Work out the finished part from the listing and answer in its coordinate system (mm). A direction names the side the tool comes from. Give positions to 0.01 mm unless a question says otherwise; leave off trailing zeros. Write each loop counter-clockwise with the first axis right and the second up, starting at its lowest first coordinate (ties: lowest second). Pieces come first, ordered by that corner, then holes. Notation, with made-up numbers: (31, 22.25) -> (56, 22.25) arc R32 cw to (56, 54.25) -> close; hole circle Ø1 at (87.5, -38.75). An arc over 180 degrees is marked (long way). Use a Markdown table: item, result. Add a question column.
Q1. For faces 1 (the face through (0, 0, 76.2)), 2 (the face through (0, -22, 12.7)), determine the directions among +Z, -Z, +X, -X, +Y, -Y from which every point of the face is accessible in a straight line to the end or side of a thin tool.
Q2. Section A-A, the plane z = 27.5 is taken. Give the vertices of the cut face in (x, y), plus the area to 3 significant figures.
Q3. Each of these flat-tipped pins is pushed along its axis until it touches: pin 1 Ø1 at (y, z) = (-29, 11) entering from +X; pin 2 Ø10 at (y, z) = (26.5, 9.5) entering from +X; pin 3 Ø2 at (x, y) = (-20.5, -16) entering from +Z; pin 4 Ø1 at (y, z) = (-16.5, 21) entering from -X. Where does it stop, or does it pass through?
Q4. Section B-B, the plane z = 67 is taken. Give the vertices of the cut face in (x, y), plus the area to 3 significant figures.
Q5. Consider line 1 (Z direction, x = -21, y = 7); line 2 (Y direction, x = 7, z = 37); line 3 (X direction, y = 5.5, z = 14). Determine where each line is inside the solid, lowest interval first.
from build123d import *

# Parameters (mm, degrees)
F0_R     = 38.1
F1_DEPTH = 12.7
F4_R     = 5.08


with BuildPart() as f1:
    # F0 (on Top) → F1 (new body)
    with BuildSketch(Plane.XY):
        Circle(F0_R)
    extrude(amount=F1_DEPTH)

    # F2 (on Front) → F3 (revolve)
    with BuildSketch(Plane.XZ):
        Polygon((0, 69.85), (0, 12.7), (16.740909, 12.7), (6.35, 69.85), (6.35, 76.2), (0, 76.2), align=None)
    revolve(axis=Axis((0, 0, 41.275), (0, 0, 1)))

    # F4
    f4_edges = [f1.edges().sort_by_distance(p)[0] for p in [
        (-38.1, 0, 12.7),
        (-38.1, 0, 0),
        (-6.35, 0, 76.2),
        (-16.740909, 0, 12.7),
    ]]
    fillet(f4_edges, radius=F4_R)


solid = f1.part
Result set:
| question | item | result |
|---|---|---|
| 1 | face 1 | +Z, +X, -X, +Y, -Y |
| 1 | face 2 | +Z |
| 2 | outline | circle Ø28.1 at (0, 0) |
| 2 | area | 620 mm2 |
| 3 | pin 1 | stops at x = 23.58 |
| 3 | pin 2 | stops at x = 31.3 |
| 3 | pin 3 | stops at z = 12.7 |
| 3 | pin 4 | passes through |
| 4 | outline | circle Ø13.74 at (0, 0) |
| 4 | area | 148 mm2 |
| 5 | line 1 | z = 0 to 12.7 |
| 5 | line 2 | y = -10.14 to 10.14 |
| 5 | line 3 | x = -16.7 to 16.7 |
